from build123d import *

# Parameters (mm, degrees)
SKETCH2_R           = 13
SKETCH2_R_2         = 10.25
BOSS_EXTRUDE1_DEPTH = 64
SKETCH3_R           = 13
BOSS_EXTRUDE2_DEPTH = 32
SKETCH4_R           = 10.25
CUT_EXTRUDE1_DEPTH  = 32
SKETCH5_R           = 10.25
CUT_EXTRUDE2_DEPTH  = 78
SKETCH6_R           = 10.75
CUT_EXTRUDE3_DEPTH  = 20
CUT_EXTRUDE4_START  = -20
SKETCH7_R           = 10.75
CUT_EXTRUDE4_DEPTH  = 20
SKETCH8_R           = 10.75
CUT_EXTRUDE5_DEPTH  = 20
FILLET1_R           = 0.2


with BuildPart() as part:
    # Sketch2 → Boss-Extrude1 (new body)
    with BuildSketch(Plane.XY):
        Circle(SKETCH2_R)
        Circle(SKETCH2_R_2, mode=Mode.SUBTRACT)
    extrude(amount=-BOSS_EXTRUDE1_DEPTH)

    # Sketch3 → Boss-Extrude2 (add)
    with BuildSketch(Plane(origin=(32, 0, 0), x_dir=(0, 0, -1), z_dir=(1, 0, 0))):
        with Locations((32, 0)):
            Circle(SKETCH3_R)
    extrude(amount=-BOSS_EXTRUDE2_DEPTH)

    # Sketch4 → Cut-Extrude1 (cut)
    with BuildSketch(Plane(origin=(32, 0, 0), x_dir=(0, 0, -1), z_dir=(1, 0, 0))):
        with Locations((32, 0)):
            Circle(SKETCH4_R)
    extrude(amount=-CUT_EXTRUDE1_DEPTH, mode=Mode.SUBTRACT)

    # Sketch5 → Cut-Extrude2 (cut)
    with BuildSketch(Plane.XY):
        Circle(SKETCH5_R)
    extrude(amount=-CUT_EXTRUDE2_DEPTH, mode=Mode.SUBTRACT)

    # Sketch6 → Cut-Extrude3 (cut)
    with BuildSketch(Plane.XY):
        Circle(SKETCH6_R)
    extrude(amount=-CUT_EXTRUDE3_DEPTH, mode=Mode.SUBTRACT)

    # Sketch7 → Cut-Extrude4 (cut)
    with BuildSketch(Plane(origin=(0, 0, -64), x_dir=(-1, 0, 0), z_dir=(0, 0, -1)).offset(CUT_EXTRUDE4_START)):
        with Locations(Location((0, 0, 0), (0, 0, 180))):
            Circle(SKETCH7_R)
    extrude(amount=CUT_EXTRUDE4_DEPTH, mode=Mode.SUBTRACT)

    # Sketch8 → Cut-Extrude5 (cut)
    with BuildSketch(Plane(origin=(32, 0, 0), x_dir=(0, 0, -1), z_dir=(1, 0, 0))):
        with Locations((32, 0)):
            Circle(SKETCH8_R)
    extrude(amount=-CUT_EXTRUDE5_DEPTH, mode=Mode.SUBTRACT)

    # Fillet1
    fillet1_edges = [part.edges().sort_by_distance(p)[0] for p in [
        (32, 0, -19),
        (-13, 0, 0),
        (-13, 0, -64),
    ]]
    fillet(fillet1_edges, radius=FILLET1_R)


solid = part.part
Geometry: final body of the model. Coordinates: model frame, mm. A direction names the side the tool comes from. Round coordinates to 2 decimals unless told otherwise and drop trailing zeros. Loops run counter-clockwise (first coordinate to the right, second up) from the corner with the lowest first, then second, coordinate; pieces in that order, holes last. Notation, with made-up numbers: (-38, 71.25) -> (-16, 71.25) arc R23 ccw to (-16, 81.25) -> close; hole circle Ø9 at (89, 55.5). An arc over 180 degrees is marked (long way). One line per question, with ' | ' between items. Start each with the question number.
1. Section C-C on z = -15. Output: boundary loops of the cut face in (x, y).
2. Line query: line 1 along Y through (x, z) = (0, -14); line 2 along Z through (x, y) = (22.5, -0.5); line 3 along Z through (x, y) = (24, -8). Output: solid intervals per line, ascending. Write a range as [from, to].
3. Set-up query: faces 1 (the face through (22.14, 3.229, -42.254)), 2 (the face through (-1.4, 10.66, -9.86)), 3 (the face through (-1.4, -10.66, -53.86)). Return all of +Z, -Z, +X, -X, +Y, -Y with unobstructed straight access to the full face (end or side cutting, diameter ignored); none if empty.
4. Mould query, pull axis Y, two halves, no side actions, for faces 4 (the face through (-12.987, 0.572, -31.555)), 5 (the face through (-7, 9, -64)), 6 (the face through (8.751, 8.643, -37.51)). Classes: pulls with the +Y half, pulls with the -Y half, needs draft (parallel to the pull), parting line crosses it, or undercut.
5. Contact query for flat-ended pins moving along their axis: pin 1 (5 mm diameter, centred on x = 27, y = 9, fed in from +Z); pin 2 (1.5 mm diameter, centred on y = 6.5, z = -25, fed in from +X); pin 3 (1 mm diameter, centred on y = 7.5, z = -14, fed in from -X); pin 4 (5 mm diameter, centred on x = -2.5, z = -21.5, fed in from +Y). Output: stop coordinate, or through.
6. Section B-B on z = -32. Output: boundary loops of the cut face in (x, y).
7. Section D-D on x = 15.5. Output: boundary loops of the cut face in (y, z), and give its area (3 significant figures).
8. Section A-A on y = 0. Count the separate pieces of the cut face and the enclosed holes in it, and give its area (3 significant figures).
Returned:
1) outline: circle Ø26 at (0, 0); hole circle Ø21.5 at (0, 0)
2) line 1: y = [-13, -10.75], [10.75, 13] | line 2: z = [-44.99, -42.74], [-21.26, -19.01] | line 3: z = [-42.25, -39.18], [-24.82, -21.75]
3) face 1: +X | face 2: +Z | face 3: -Z
4) face 4: parting line crosses it | face 5: needs draft | face 6: undercut
5) pin 1: stops at z = -20.74 | pin 2: stops at x = 12 | pin 3: stops at x = -10.95 | pin 4: stops at y = 13
6) outline: (0, -13) -> (31.8, -13) arc R0.2 ccw to (32, -12.8) -> (32, -10.75) -> (12, -10.75) -> (12, -10.25) -> (0, -10.25) arc R10.25 cw to (0, 10.25) -> (12, 10.25) -> (12, 10.75) -> (32, 10.75) -> (32, 12.8) arc R0.2 ccw to (31.8, 13) -> (0, 13) arc R13 ccw to start
7) outline: circle Ø26 at (0, -32); hole circle Ø21.5 at (0, -32) | area: 168 mm2
8) separate pieces: 3 | enclosed holes: 0 | area: 340 mm2
